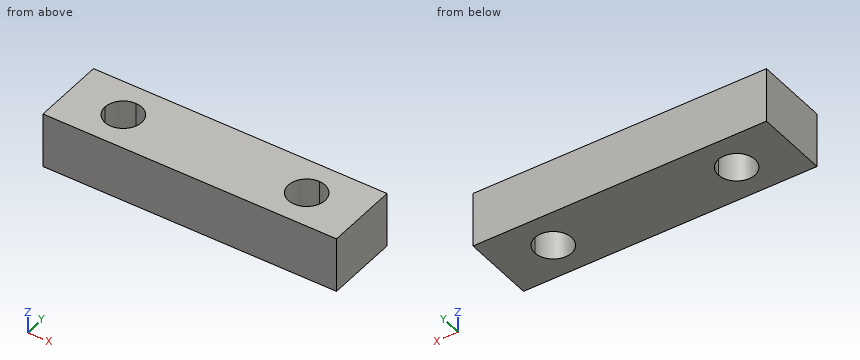
```python
from build123d import *

# Parameters (mm, degrees)
F0_W     = 2032
F0_H     = 381
F1_DEPTH = 508
F3_DEPTH = 508


with BuildPart() as f1:
    # F0 (on Front) → F1 (new body)
    with BuildSketch(Plane.XZ):
        with Locations((-1016, 190.5)):
            Rectangle(F0_W, F0_H)
    extrude(amount=F1_DEPTH)

    # F2 (on face) → F3 (cut)
    with BuildSketch(Plane.XY.offset(381)):
        with BuildLine():
            ThreePointArc((-1524, -254), (-1561.197439, -164.197439), (-1651, -127))
            Line((-1651, -127), (-1651, -254))
            Line((-1651, -254), (-1778, -254))
            ThreePointArc((-1778, -254), (-1651, -381), (-1524, -254))
        make_face()
        with BuildLine():
            Line((-1651, -254), (-1651, -127))
            ThreePointArc((-1651, -127), (-1740.802561, -164.197439), (-1778, -254))
            Line((-1778, -254), (-1651, -254))
        make_face()
        with BuildLine():
            ThreePointArc((-254, -254), (-291.197439, -164.197439), (-381, -127))
            Line((-381, -127), (-381, -254))
            Line((-381, -254), (-254, -254))
        make_face()
        with BuildLine():
            Line((-381, -254), (-381, -127))
            ThreePointArc((-381, -127), (-470.802561, -343.802561), (-254, -254))
            Line((-254, -254), (-381, -254))
        make_face()
    extrude(amount=-F3_DEPTH, mode=Mode.SUBTRACT)


solid = f1.part
```
The model under review builds one solid part; all positions refer to its coordinate system, in mm. Round coordinates to 2 decimals unless told otherwise and drop trailing zeros. Order: outer loops, then holes, each group sorted by start corner. A loop starts at its lowest first (then second) coordinate and runs counter-clockwise, first axis right, second up.
(1) Take a section at A-A, the plane z = 161.5. State the section outline as (x, y) points.
Working result:
outline: (-2032, -508) - (0, -508) - (0, 0) - (-2032, 0) - close; hole (-1778, -254) arc R127 ccw (long way) to (-1651, -127) arc R127 ccw to start; hole circle Ø254 at (-381, -254)
(2) Take a section at B-B, the plane y = -175. State the section outline as (x, z) points.
Working result:
outline: (-2032, 0) - (-1750.44, 0) - (-1750.44, 381) - (-2032, 381) - close; (-1551.56, 0) - (-480.44, 0) - (-480.44, 381) - (-1551.56, 381) - close; (-281.56, 0) - (0, 0) - (0, 381) - (-281.56, 381) - close
(3) Take a section at C-C, the plane y = -359. State the section outline as (x, z) points, plus the area to 3 significant figures.
Working result:
outline: (-2032, 0) - (-1722.44, 0) - (-1722.44, 381) - (-2032, 381) - close; (-1579.56, 0) - (-452.44, 0) - (-452.44, 381) - (-1579.56, 381) - close; (-309.56, 0) - (0, 0) - (0, 381) - (-309.56, 381) - close
area: 665,000 mm2
(4) Wall thickness on L1, parallel to X at y = -254, z = 156.5; L2, parallel to Y at x = -381, z = 302; L3, parallel to X at y = -204, z = 23: over which ranges is each line inside the solid? List them lowest first.
Working result:
L1: x = -2032 to -1778, -1524 to -508, -254 to 0
L2: y = -508 to -381, -127 to 0
L3: x = -2032 to -1767.74, -1534.26 to -497.74, -264.26 to 0
